```python
from build123d import *
from build123d.topology import SkipClean

# Parameters (mm, degrees)
SKETCH1_R           = 7.5
BOSS_EXTRUDE1_DEPTH = 1.85
BOSS_EXTRUDE2_START = 8
BOSS_EXTRUDE2_DEPTH = 8
SKETCH4_R           = 3.5
CUT_EXTRUDE1_DEPTH  = 14.285330256
SKETCH5_R           = 4
SKETCH5_R_2         = 3.5
BOSS_EXTRUDE3_DEPTH = 7
SKETCH6_R           = 4
BOSS_EXTRUDE4_DEPTH = 7
SKETCH7_R           = 4
BOSS_EXTRUDE5_DEPTH = 2


with BuildPart() as part:
    # Sketch1 → Boss-Extrude1 (new body)
    with BuildSketch(Plane(origin=(0, 0, 0), x_dir=(1, 0, 0), z_dir=(0, 1, 0))):
        with Locations(Location((0, 0, 0), (0, 0, 270))):
            Circle(SKETCH1_R)
    extrude(amount=BOSS_EXTRUDE1_DEPTH)

    # Sketch2 → Boss-Extrude2 (add)
    with SkipClean():  # the faces are left unmerged after this step: merging them gives an invalid solid
        with BuildSketch(Plane.XZ.offset(BOSS_EXTRUDE2_START)):
            with BuildLine():
                Line((2.5, 7.071067812), (2.5, -7.071067812))
                ThreePointArc((2.5, -7.071067812), (7.5, 0), (2.5, 7.071067812))
            make_face()
        extrude(amount=-BOSS_EXTRUDE2_DEPTH)

    # Sketch4 → Cut-Extrude1 (cut, through all)
    with SkipClean():  # the faces are left unmerged after this step: merging them gives an invalid solid
        with BuildSketch(Plane(origin=(0, 0, 0), x_dir=(0, 0, -1), z_dir=(1, 0, 0))):
            with Locations(Location((0, -4, 0), (0, 0, 270))):
                Circle(SKETCH4_R)
        extrude(amount=CUT_EXTRUDE1_DEPTH, mode=Mode.SUBTRACT)

    # Sketch5 → Boss-Extrude3 (add)
    with SkipClean():  # the faces are left unmerged after this step: merging them gives an invalid solid
        with BuildSketch(Plane.ZY.offset(-2.5)):
            with Locations((0, -4)):
                Circle(SKETCH5_R)
            with Locations((0, -4)):
                Circle(SKETCH5_R_2, mode=Mode.SUBTRACT)
        extrude(amount=-BOSS_EXTRUDE3_DEPTH)

    # Sketch6 → Boss-Extrude4 (add)
    with SkipClean():  # the faces are left unmerged after this step: merging them gives an invalid solid
        with BuildSketch(Plane(origin=(0, 1.85, 0), x_dir=(1, 0, 0), z_dir=(0, 1, 0))):
            with Locations(Location((0, 0, 0), (0, 0, 270))):
                Circle(SKETCH6_R)
        extrude(amount=BOSS_EXTRUDE4_DEPTH)

    # Sketch7 → Boss-Extrude5 (add)
    with SkipClean():  # the faces are left unmerged after this step: merging them gives an invalid solid
        with BuildSketch(Plane(origin=(9.5, 0, 0), x_dir=(0, 0, -1), z_dir=(1, 0, 0))):
            with Locations(Location((0, -4, 0), (0, 0, 270))):
                Circle(SKETCH7_R)
        extrude(amount=BOSS_EXTRUDE5_DEPTH)


solid = part.part
```
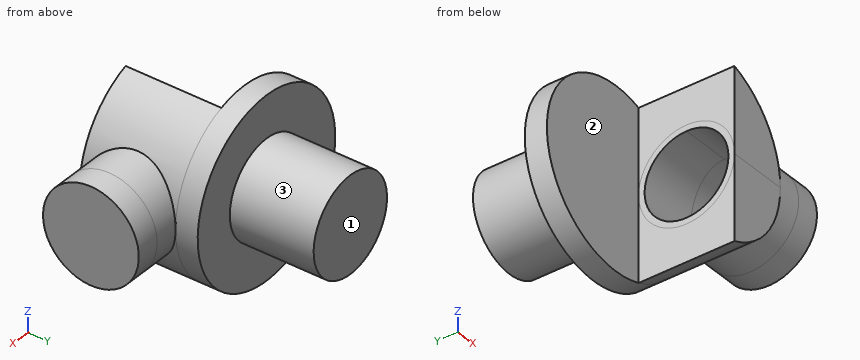
Verification items for the finished model (mm, model axes). Face numbers are marked on the shaded views. A direction names the side the tool comes from. Coordinates: 2 decimals unless noted, no trailing zeros. Loops run counter-clockwise (first coordinate to the right, second up) from the corner with the lowest first, then second, coordinate; pieces in that order, holes last. Notation, with made-up numbers: (26, -5) -> (79, -5) arc R8 ccw to (79, 0) -> close; hole circle Ø10 at (-34, 12.25). An arc over 180 degrees is marked (long way). Answer in a Markdown table with one row per item. Add a question column.
1. Material ranges on probe 1 along Z at (x, y) = (8, -4); probe 2 along X at (y, z) = (-1, 0.5); probe 3 along Z at (x, y) = (6.75, -3), recorded low to high. Write a range as [from, to].
2. Section check A-A, the plane z = -1.25. Enter the section's corners in (x, y).
3. Section check D-D, the plane x = 3.25. Enter the section's corners in (y, z), then the cut area to 3 significant figures.
4. Section check B-B, the plane y = -5.5. Enter the section's corners in (x, z).
5. Access from +Z, -Z, +X, -X, +Y, -Y to the whole of each face (thin tool, end or side, straight path). Record for the marked faces 1, 2 and 3.
6. Depth check by flat-ended pin: P1, Ø9, axis at y = -6, z = -2, coming from the -X side; P2, Ø3, axis at x = -2, z = -1.5, coming from the -Y side; P3, Ø2, axis at y = -5.5, z = 0.5, coming from the -X side; P4, Ø6, axis at x = -2.5, y = -5.5, coming from the -Z side. Enter the tip coordinate at first touch or a pass-through.
7. Section check C-C, the plane x = 0. Enter the section's corners in (y, z), then the cut area to 4 significant figures.
Derived:
| question | item | result |
|---|---|---|
| 1 | probe 1 | z = [-4, -3.5], [3.5, 4] |
| 1 | probe 2 | x = [9.5, 11.5] |
| 1 | probe 3 | z = [-3.87, -3.35], [3.35, 3.87] |
| 2 | outline | (-7.4, 0) -> (2.5, 0) -> (2.5, -0.73) -> (9.5, -0.73) -> (9.5, -7.27) -> (2.5, -7.27) -> (2.5, -8) -> (7.4, -8) -> (7.4, -7.8) -> (11.5, -7.8) -> (11.5, -0.2) -> (7.4, -0.2) -> (7.4, 1.85) -> (3.8, 1.85) -> (3.8, 8.85) -> (-3.8, 8.85) -> (-3.8, 1.85) -> (-7.4, 1.85) -> close |
| 3 | outline | (-8, -6.76) -> (1.85, -6.76) -> (1.85, -2.33) -> (8.85, -2.33) -> (8.85, 2.33) -> (1.85, 2.33) -> (1.85, 6.76) -> (-8, 6.76) -> close; hole circle Ø7 at (-4, 0) |
| 3 | area | 127 mm² |
| 4 | outline | (2.5, -7.07) arc R7.5 ccw to (6.52, -3.71) -> (11.5, -3.71) -> (11.5, 3.71) -> (6.52, 3.71) arc R7.5 ccw to (2.5, 7.07) -> (2.5, 3.16) -> (9.5, 3.16) -> (9.5, -3.16) -> (2.5, -3.16) -> close |
| 5 | face 1 | +Z, -Z, +X, -X, +Y |
| 5 | face 2 | +Z, -Z, -X, -Y |
| 5 | face 3 | +Y |
| 6 | P1 | stops at x = 2.5 |
| 6 | P2 | stops at y = 0 |
| 6 | P3 | stops at x = 9.5 |
| 6 | P4 | passes through |
| 7 | outline | (0, -7.5) -> (1.85, -7.5) -> (1.85, -4) -> (8.85, -4) -> (8.85, 4) -> (1.85, 4) -> (1.85, 7.5) -> (0, 7.5) -> close |
| 7 | area | 83.75 mm² |
